```python
from build123d import *

# Parameters (mm, degrees)
SKETCH1_W           = 150
SKETCH1_H           = 150
BOSS_EXTRUDE1_DEPTH = 110
SKETCH3_W           = 126
SKETCH3_H           = 126
CUT_EXTRUDE1_DEPTH  = 98
SKETCH4_R           = 1.7
SKETCH4_R_2         = 25
CUT_EXTRUDE2_DEPTH  = 239.956062907
CUT_EXTRUDE3_DEPTH  = 239.956062907
CUT_EXTRUDE4_START  = 150
CUT_EXTRUDE4_DEPTH  = 12
SKETCH5_R           = 4
SKETCH5_R_2         = 10
CUT_EXTRUDE5_DEPTH  = 12


with BuildPart() as part:
    # Sketch1 → Boss-Extrude1 (new body)
    with BuildSketch(Plane(origin=(0, 0, 0), x_dir=(1, 0, 0), z_dir=(0, 1, 0))):
        with Locations((75, 75)):
            Rectangle(SKETCH1_W, SKETCH1_H)
    extrude(amount=BOSS_EXTRUDE1_DEPTH)

    # Sketch3 → Cut-Extrude1 (cut)
    with BuildSketch(Plane.XZ):
        with Locations((75, -75)):
            Rectangle(SKETCH3_W, SKETCH3_H)
    extrude(amount=-CUT_EXTRUDE1_DEPTH, mode=Mode.SUBTRACT)

    # Sketch4 → Cut-Extrude2 (cut, through all)
    with BuildSketch(Plane(origin=(0, 110, 0), x_dir=(1, 0, 0), z_dir=(0, 1, 0))):
        with Locations(Location((75, 130, 0), (0, 0, 270))):
            Circle(SKETCH4_R)
        with Locations(Location((130, 75, 0), (0, 0, 270))):
            Circle(SKETCH4_R)
        with Locations(Location((75, 20, 0), (0, 0, 270))):
            Circle(SKETCH4_R)
        with Locations(Location((20, 75, 0), (0, 0, 270))):
            Circle(SKETCH4_R)
        with Locations(Location((75, 75, 0), (0, 0, 270))):
            Circle(SKETCH4_R_2)
    extrude(amount=-CUT_EXTRUDE2_DEPTH, mode=Mode.SUBTRACT)

    # Sketch6 → Cut-Extrude3 (cut, through all)
    with BuildSketch(Plane.ZY):
        with BuildLine():
            Line((-90, 10), (-60, 10))
            ThreePointArc((-60, 10), (-48.819660113, 7.360679775), (-40, 0))
            Line((-40, 0), (-110, 0))
            ThreePointArc((-110, 0), (-101.180339887, 7.360679775), (-90, 10))
        make_face()
    extrude(amount=-CUT_EXTRUDE3_DEPTH, mode=Mode.SUBTRACT)

    # Sketch7 → Cut-Extrude4 (cut)
    with BuildSketch(Plane(origin=(0, 0, 0), x_dir=(-1, 0, 0), z_dir=(0, 0, -1)).offset(CUT_EXTRUDE4_START)):
        with BuildLine():
            Line((-90, 10), (-60, 10))
            ThreePointArc((-60, 10), (-48.819660113, 7.360679775), (-40, 0))
            Line((-40, 0), (-110, 0))
            ThreePointArc((-110, 0), (-101.180339887, 7.360679775), (-90, 10))
        make_face()
    extrude(amount=-CUT_EXTRUDE4_DEPTH, mode=Mode.SUBTRACT)

    # Sketch5 → Cut-Extrude5 (cut)
    with BuildSketch(Plane.XY):
        with Locations((40, 65)):
            Circle(SKETCH5_R)
        with Locations((75, 45)):
            Circle(SKETCH5_R_2)
        with Locations((110, 65)):
            Circle(SKETCH5_R)
        with Locations((40, 20)):
            Circle(SKETCH5_R)
        with Locations((110, 20)):
            Circle(SKETCH5_R)
    extrude(amount=-CUT_EXTRUDE5_DEPTH, mode=Mode.SUBTRACT)


solid = part.part
```
Input: part model. Units: mm. Frame: model coordinates. A direction names the side the tool comes from. Coordinates: 2 decimals unless noted, no trailing zeros. Loops run counter-clockwise (first coordinate to the right, second up) from the corner with the lowest first, then second, coordinate; pieces in that order, holes last.
Q1. Contact query for flat-ended pins moving along their axis: pin 1 (9.5 mm diameter, centred on x = 144.5, z = -76, fed in from -Y); pin 2 (6.5 mm diameter, centred on x = 110, y = 65, fed in from +Z); pin 3 (3 mm diameter, centred on x = 20, z = -75, fed in from -Y). Output: stop coordinate, or through.
Results are:
pin 1: stops at y = 10
pin 2: stops at z = -138
pin 3: passes through
Q2. Section D-D, the plane y = 40. Return the cut outline in (x, z), and give its area (3 significant figures).
Results are:
outline: (0, -150) - (150, -150) - (150, 0) - (83.66, 0) - (83.66, -12) - (138, -12) - (138, -138) - (12, -138) - (12, -12) - (66.34, -12) - (66.34, 0) - (0, 0) - close
area: 6,420 mm2
Q3. Set-up query: faces 1 (the cylindrical face through (37.05, 22.7, -5.92)), 2 (the cylindrical face through (101.3, 7.3, -144.1)), 3 (the cylindrical face through (143.9, 7.3, -101.3)), 4 (the flat face through (12, 48, -76)). Return all of +Z, -Z, +X, -X, +Y, -Y with unobstructed straight access to the full face (end or side cutting, diameter ignored); none if empty.
Results are:
face 1: +Z
face 2: -Z, -Y
face 3: +X, -X, -Y
face 4: -Y
Q4. Line query: line 1 along Y through (x, z) = (40, -3); line 2 along X through (y, z) = (103.5, -75); line 3 along Z through (x, y) = (95, 83.5). Output: solid intervals per line, ascending.
Results are:
line 1: y = 0 to 16, 24 to 61, 69 to 110
line 2: x = 0 to 18.3, 21.7 to 50, 100 to 128.3, 131.7 to 150
line 3: z = -150 to -138, -12 to 0
Q5. Section A-A, the plane y = 101. Return the cut outline in (x, z), and give its area (3 significant figures).
Results are:
outline: (0, -150) - (150, -150) - (150, 0) - (0, 0) - close; hole circle Ø3.4 at (20, -75); hole circle Ø50 at (75, -75); hole circle Ø3.4 at (75, -130); hole circle Ø3.4 at (75, -20); hole circle Ø3.4 at (130, -75)
area: 20,500 mm2
Q6. Mould query, pull axis Y, two halves, no side actions, for faces 5 (the flat face through (57, 110, -93)), 6 (the flat face through (46, 98, -74)), 7 (the cylindrical face through (67, 39, -6)), 8 (the flat face through (74, 48, -138)). Classes: +Y half, -Y half, draft (parallel to the pull), parting line (faces both ways), or undercut.
Results are:
face 5: +Y half
face 6: -Y half
face 7: undercut
face 8: draft
Q7. Section C-C, the plane y = 65. Return the cut outline in (x, z).
Results are:
outline: (0, -150) - (150, -150) - (150, 0) - (114, 0) - (114, -12) - (138, -12) - (138, -138) - (12, -138) - (12, -12) - (36, -12) - (36, 0) - (0, 0) - close; (44, -12) - (106, -12) - (106, 0) - (44, 0) - close
Q8. Section B-B, the plane x = 135. Return the cut outline in (y, z), and give its area (3 significant figures).
Results are:
outline: (0, -150) - (110, -150) - (110, 0) - (0, 0) - (0, -12) - (98, -12) - (98, -138) - (0, -138) - close
area: 4,150 mm2
